```python
from build123d import *

# Parameters (mm, degrees)
CROQUIS1_R              = 2.5
CROQUIS1_R_2            = 1
SALIENTE_EXTRUIR1_DEPTH = 1
CROQUIS2_R              = 1
SALIENTE_EXTRUIR2_DEPTH = 6
VACIADO2_T              = -0.1


with BuildPart() as part:
    # Croquis1 → Saliente-Extruir1 (new body)
    with BuildSketch(Plane.XY):
        Circle(CROQUIS1_R)
        Circle(CROQUIS1_R_2, mode=Mode.SUBTRACT)
    extrude(amount=SALIENTE_EXTRUIR1_DEPTH)



with BuildPart() as body_2:
    # Croquis2 → Saliente-Extruir2 (new body)
    with BuildSketch(Plane.XY.offset(1)):
        Circle(CROQUIS2_R)
    extrude(amount=SALIENTE_EXTRUIR2_DEPTH)

    # Vaciado2
    vaciado2_openings = [body_2.faces().sort_by_distance(p)[0] for p in [
        (0, 0, 7),
        (0, 0, 1),
    ]]
    offset(amount=VACIADO2_T, openings=vaciado2_openings, kind=Kind.INTERSECTION)


with BuildPart() as part_1:
    add(part.part)

    add(body_2.part)  # Revoluci_n2 merges body 2
    # Croquis3 → Revoluci_n2 (revolve)
    with BuildSketch(Plane(origin=(0, 0, 0), x_dir=(0, 0, -1), z_dir=(1, 0, 0)), mode=Mode.PRIVATE) as revoluci_n2_sk:
        with BuildLine():
            Line((-1, 2.5), (-1, 1))
            Line((-1, 1), (-1.517000999, 1))
            add(Edge.make_bspline(
                [(-1.517000999, 1), (-1.132819845, 1.729659773), (-1, 2.5)],
                knots=[0, 0, 0, 1, 1, 1], degree=2))
        make_face()
    revolve(revoluci_n2_sk.sketch.rotate(Axis((0, 0, 7.040846827), (0, 0, -1)), 90), axis=Axis((0, 0, 7.040846827), (0, 0, -1)))


solid = part_1.part
```
Input: part model. Units: mm. Frame: model coordinates. Round coordinates to 2 decimals unless told otherwise and drop trailing zeros. Order: outer loops, then holes, each group sorted by start corner. A loop starts at its lowest first (then second) coordinate and runs counter-clockwise, first axis right, second up. Notation, with made-up numbers: (84, -10) - (141, -10) arc R19 cw to (141, 26) - close; hole circle Ø3 at (34.5, 22.5). An arc over 180 degrees is marked (long way). Answer in a Markdown table with one row per item.
Item 1: Section query A-A (z = 6). Return the cut outline in (x, y).
Model answer:
| item | result |
|---|---|
| outline | circle Ø2 at (0, 0); hole circle Ø1.8 at (0, 0) |
Item 2: Line query: line 1 (Y direction, x = 0, z = 0.7); line 2 (Z direction, x = 0.15, y = -1.05); line 3 (Z direction, x = -1, y = -0.8). Output: solid intervals per line, ascending.
Model answer:
| item | result |
|---|---|
| line 1 | y = -2.5 to -1, 1 to 2.5 |
| line 2 | z = 0 to 1.49 |
| line 3 | z = 0 to 1.38 |
Item 3: Pin query (flat end, axial travel): pin 1 (3 mm diameter, centred on x = 1, z = 3, fed in from +Y); pin 2 (2 mm diameter, centred on y = 1, z = 1.5, fed in from -X). Return the tip coordinate at first contact, or that it passes through.
Model answer:
| item | result |
|---|---|
| pin 1 | stops at y = 1 |
| pin 2 | stops at x = -2.5 |
Item 4: Mould query, pull axis Y, two halves, no side actions, for faces 1 (the flat face through (1, -1, 0)), 2 (the cylindrical face through (-0.54, -2.44, 0.49)), 3 (the cylindrical face through (-0.217, -0.976, 0.493)). Classes: released by +Y, released by -Y, zero draft, split by the parting line, or undercut.
Model answer:
| item | result |
|---|---|
| face 1 | zero draft |
| face 2 | split by the parting line |
| face 3 | undercut |
